CAD build for the part. Positions are in the model's coordinates, mm. A direction names the side the tool comes from. Round coordinates to 2 decimals unless told otherwise and drop trailing zeros. Order: outer loops, then holes, each group sorted by start corner. A loop starts at its lowest first (then second) coordinate and runs counter-clockwise, first axis right, second up. Notation, with made-up numbers: M 21.5,26.25 L 63.5,26.25 A20 cw 63.5,30.25 Z; hole C 40.25,-3.5 d8. An arc over 180 degrees is marked long. Answer as a JSON object with one key per item and string values.
```python
from build123d import *


with BuildPart() as part:
    # Sketch1 → Revolve1 (revolve)
    with BuildSketch(Plane.XY, mode=Mode.PRIVATE) as revolve1_sk:
        Polygon((0, 4), (5.89, 4), (5.89, 9), (4.730911447, 9), (4.730911447, 24.74), (5.89, 24.74), (5.89, 27.74), (0, 27.74), align=None)
    revolve1 = revolve(revolve1_sk.sketch.rotate(Axis((0, 0, 0), (1, 0, 0)), 90), axis=Axis((0, 0, 0), (1, 0, 0)))

    # Sketch2 → Cut-Revolve1 (revolve, cut)
    with BuildSketch(Plane.XY, mode=Mode.PRIVATE) as cut_revolve1_sk:
        Polygon((0, 19.74), (1.977829822, 19.74), (4.889591697, 27.74), (0, 27.74), align=None)
    cut_revolve1 = revolve(cut_revolve1_sk.sketch.rotate(Axis((0, 0, 0), (1, 0, 0)), 90), axis=Axis((0, 0, 0), (1, 0, 0)), mode=Mode.SUBTRACT)

    # Mirror1: Revolve1, Cut-Revolve1 across plane
    add(revolve1.mirror(Plane(origin=(0, 27.74, 0), x_dir=(0, 0, 1), z_dir=(1, 0, 0))))
    add(cut_revolve1.mirror(Plane(origin=(0, 27.74, 0), x_dir=(0, 0, 1), z_dir=(1, 0, 0))), mode=Mode.SUBTRACT)


solid = part.part
```
Item 1: Saw through at C-C on x = 1. List the corners of the cut face in (y, z), and give its area (3 significant figures).
Worked answers:
{"outline": "C 0,0 d39.48; hole C 0,0 d8", "area": "1,170 mm2"}
Item 2: Two-plate mould, pull along Y, no slides. Class faces 6 (the cylindrical face through (5.319, 21.949, 11.416)), 7 (the flat face through (5.89, 4, -2)), 8 (the conical face through (-2.16, -6.08, 19.31)), 9 (the cylindrical face through (-5.302, -6.083, -6.633)): released by +Y, released by -Y, zero draft, split by the parting line, or undercut.
Worked answers:
{"face 6": "undercut", "face 7": "zero draft", "face 8": "split by the parting line", "face 9": "undercut"}
Item 3: 3-axis set-ups, long thin cutter, end or side, ignore diameter. For faces 1 (the flat face through (4.731, 11, 0)), 2 (the conical face through (2.16, -6.08, 19.31)), 3 (the cylindrical face through (-5.319, 21.949, 11.416)), 4 (the flat face through (5.89, 0, 25)), 5 (the flat face through (-5.89, 4, -2)): which of +Z, -Z, +X, -X, +Y, -Y reach the whole face in a straight line?
Worked answers:
{"face 1": "+X", "face 2": "none", "face 3": "-X", "face 4": "+Z, -Z, +X, +Y, -Y", "face 5": "+Z, -Z, -X, +Y, -Y"}
Item 4: Drop flat-ended pins along their axis: pin 1 Ø3 at (x, z) = (4, 2) entering from -Y; pin 2 Ø4 at (x, y) = (-4.5, 15) entering from -Z; pin 3 Ø2 at (x, z) = (1, -4.5) entering from -Y. Give the stop position or say it passes through.
Worked answers:
{"pin 1": "stops at y = -27.73", "pin 2": "stops at z = -24.48", "pin 3": "stops at y = -19.43"}
Item 5: Wall check: line 1 along Y through (x, z) = (-5.45, 0); line 2 along Y through (x, z) = (-1.75, 0); line 3 along X through (y, z) = (-19, 2.5). Give the ranges that are in metal, low to high. Write a range as [from, to].
Worked answers:
{"line 1": "y = [-27.74, -24.74], [-9, -4], [4, 9], [24.74, 27.74]", "line 2": "y = [-19.74, -4], [4, 19.74]", "line 3": "x = [-4.73, 4.73]"}
